from build123d import *

# Parameters (mm, degrees)
SKETCH1_R             = 20
SKETCH1_R_2           = 15
BOSS_EXTRUDE1_DEPTH   = 15
SKETCH1_R_3           = 40
SKETCH1_R_4           = 16
BOSS_EXTRUDE1_2_DEPTH = 15
BOSS_EXTRUDE1_3_DEPTH = 15
SKETCH1_3_R           = 15
BOSS_EXTRUDE2_DEPTH   = 5


with BuildPart() as part:
    # Sketch1 → Boss-Extrude1 (new, symmetric)
    with BuildSketch(Plane.XY):
        with Locations((-70, 0)):
            Circle(SKETCH1_R)
        with Locations((-70, 0)):
            Circle(SKETCH1_R_2, mode=Mode.SUBTRACT)
    extrude(amount=BOSS_EXTRUDE1_DEPTH, both=True)



with BuildPart() as body_2:
    # Sketch1 → Boss-Extrude1 2 (new, symmetric)
    with BuildSketch(Plane.XY):
        Circle(SKETCH1_R_3)
        Circle(SKETCH1_R_4, mode=Mode.SUBTRACT)
        with BuildLine():
            ThreePointArc((26.090759323, 18.527608533), (16, 27.712812921), (3, 31.859064644))
            Line((3, 31.859064644), (3, 20.784609691))
            ThreePointArc((3, 20.784609691), (10.5, 18.186533479), (16.5, 12.990381057))
            Line((16.5, 12.990381057), (26.090759323, 18.527608533))
        make_face(mode=Mode.SUBTRACT)
        with BuildLine():
            ThreePointArc((29.090759323, -13.331456111), (32, 0), (29.090759323, 13.331456111))
            Line((29.090759323, 13.331456111), (19.5, 7.794228634))
            ThreePointArc((19.5, 7.794228634), (21, 0), (19.5, -7.794228634))
            Line((19.5, -7.794228634), (29.090759323, -13.331456111))
        make_face(mode=Mode.SUBTRACT)
        with BuildLine():
            ThreePointArc((3, -31.859064644), (16, -27.712812921), (26.090759323, -18.527608533))
            Line((26.090759323, -18.527608533), (16.5, -12.990381057))
            ThreePointArc((16.5, -12.990381057), (10.5, -18.186533479), (3, -20.784609691))
            Line((3, -20.784609691), (3, -31.859064644))
        make_face(mode=Mode.SUBTRACT)
        with BuildLine():
            ThreePointArc((-26.090759323, -18.527608533), (-16, -27.712812921), (-3, -31.859064644))
            Line((-3, -31.859064644), (-3, -20.784609691))
            ThreePointArc((-3, -20.784609691), (-10.5, -18.186533479), (-16.5, -12.990381057))
            Line((-16.5, -12.990381057), (-26.090759323, -18.527608533))
        make_face(mode=Mode.SUBTRACT)
        with BuildLine():
            ThreePointArc((-29.090759323, 13.331456111), (-32, 0), (-29.090759323, -13.331456111))
            Line((-29.090759323, -13.331456111), (-19.5, -7.794228634))
            ThreePointArc((-19.5, -7.794228634), (-21, 0), (-19.5, 7.794228634))
            Line((-19.5, 7.794228634), (-29.090759323, 13.331456111))
        make_face(mode=Mode.SUBTRACT)
        with BuildLine():
            ThreePointArc((-3, 31.859064644), (-16, 27.712812921), (-26.090759323, 18.527608533))
            Line((-26.090759323, 18.527608533), (-16.5, 12.990381057))
            ThreePointArc((-16.5, 12.990381057), (-10.5, 18.186533479), (-3, 20.784609691))
            Line((-3, 20.784609691), (-3, 31.859064644))
        make_face(mode=Mode.SUBTRACT)
    extrude(amount=BOSS_EXTRUDE1_2_DEPTH, both=True)


with BuildPart() as body_3:
    # Sketch1 → Boss-Extrude1 3 (new, symmetric)
    with BuildSketch(Plane.XY):
        with Locations((70, 0)):
            Circle(SKETCH1_R)
        with Locations((70, 0)):
            Circle(SKETCH1_R_2, mode=Mode.SUBTRACT)
    extrude(amount=BOSS_EXTRUDE1_3_DEPTH, both=True)


with BuildPart() as part_1:
    add(part.part)

    add(body_2.part)  # Boss-Extrude2 merges body 2

    add(body_3.part)  # Boss-Extrude2 merges body 3
    # Sketch1_3 → Boss-Extrude2 (add, symmetric)
    # profile 1 of 2: a face of its own
    with BuildSketch(Plane.XY):
        with BuildLine():
            ThreePointArc((-89.071294105, 6.023764702), (-50, 0), (-89.071294105, -6.023764702))
            Line((-89.071294105, -6.023764702), (-70.02485881, -66.324952937))
            ThreePointArc((-70.02485881, -66.324952937), (-46.6282273, -80.727545655), (-29.002885891, -59.651863383))
            ThreePointArc((-29.002885891, -59.651863383), (-22.168588856, -44.262528341), (-6.003756239, -39.546869801))
            ThreePointArc((-6.003756239, -39.546869801), (-40, 0), (-6.003756239, 39.546869801))
            ThreePointArc((-6.003756239, 39.546869801), (-22.168588856, 44.262528341), (-29.002885891, 59.651863383))
            ThreePointArc((-29.002885891, 59.651863383), (-46.6282273, 80.727545655), (-70.02485881, 66.324952937))
            Line((-70.02485881, 66.324952937), (-89.071294105, 6.023764702))
        make_face()
        with Locations((-50, -60)):
            Circle(SKETCH1_3_R, mode=Mode.SUBTRACT)
        with Locations((-50, 60)):
            Circle(SKETCH1_3_R, mode=Mode.SUBTRACT)
    # profile 2 of 2: a face of its own
    with BuildSketch(Plane.XY):
        with BuildLine():
            ThreePointArc((6.003756239, 39.546869801), (40, 0), (6.003756239, -39.546869801))
            ThreePointArc((6.003756239, -39.546869801), (22.168588856, -44.262528341), (29.002885891, -59.651863383))
            ThreePointArc((29.002885891, -59.651863383), (46.6282273, -80.727545655), (70.02485881, -66.324952937))
            Line((70.02485881, -66.324952937), (89.071294105, -6.023764702))
            ThreePointArc((89.071294105, -6.023764702), (50, 0), (89.071294105, 6.023764702))
            Line((89.071294105, 6.023764702), (70.02485881, 66.324952937))
            ThreePointArc((70.02485881, 66.324952937), (46.6282273, 80.727545655), (29.002885891, 59.651863383))
            ThreePointArc((29.002885891, 59.651863383), (22.168588856, 44.262528341), (6.003756239, 39.546869801))
        make_face()
        with Locations((50, -60)):
            Circle(SKETCH1_3_R, mode=Mode.SUBTRACT)
        with Locations((50, 60)):
            Circle(SKETCH1_3_R, mode=Mode.SUBTRACT)
    extrude(amount=BOSS_EXTRUDE2_DEPTH, both=True)


solid = part_1.part
Source: CAD feature listing. Evaluate the final solid. Frame: model axes, mm. A direction names the side the tool comes from. Coordinates: 2 decimals unless noted, no trailing zeros. Loops run counter-clockwise (first coordinate to the right, second up) from the corner with the lowest first, then second, coordinate; pieces in that order, holes last. Notation, with made-up numbers: (10.5, 65) - (36.5, 65) arc R21 cw to (36.5, 70) - close; hole circle Ø10 at (-37.5, 27). An arc over 180 degrees is marked (long way). One line per item, written item: value. Start each with the question number.
1. Mould query, pull axis Y, two halves, no side actions, for faces 1 (the flat face through (73, 15, 15)), 2 (the cylindrical face through (-21, 0, 0)), 3 (the flat face through (-79.681, -35.752, -0.07)). Classes: pulls with the +Y half, pulls with the -Y half, needs draft (parallel to the pull), parting line crosses it, or undercut.
2. Section B-B (y = -69.5). Return the cut outline in (x, z), and give its area (3 significant figures).
3. Section A-A (x = 0). Return the cut outline in (y, z).
4. Section D-D (y = -47). Return the cut outline in (x, z), and give its area (3 significant figures).
5. Ray query, L1, parallel to Y at x = 50, z = 0.5; L2, parallel to X at y = 25.5, z = -1.5; L3, parallel to Y at x = 52, z = -1.75. Return the intervals inside material, ascending.
6. Contact query for flat-ended pins moving along their axis: P1, Ø5.5, axis at y = -26, z = 0.5, coming from the -X side; P2, Ø2, axis at y = -14, z = -6.5, coming from the +X side; P3, Ø1.5, axis at x = 26.5, y = -49.5, coming from the +Z side; P4, Ø18, axis at x = 70, y = 0, coming from the +Z side. Output: stop coordinate, or through.
7. Set-up query: faces 4 (the flat face through (-21.23, -15.72, 0.21)), 5 (the flat face through (17, 1, -15)), 6 (the flat face through (47, 6, -5)). Return all of +Z, -Z, +X, -X, +Y, -Y with unobstructed straight access to the full face (end or side cutting, diameter ignored); none if empty.
8. Section C-C (y = -25.5). Return the cut outline in (x, z), and give its area (3 significant figures).
Verdict:
1. face 1: needs draft
1. face 2: undercut
1. face 3: pulls with the -Y half
2. outline: (-68.73, -5) - (-61.61, -5) - (-61.61, 5) - (-68.73, 5) - close; (-38.39, -5) - (-31.27, -5) - (-31.27, 5) - (-38.39, 5) - close; (31.27, -5) - (38.39, -5) - (38.39, 5) - (31.27, 5) - close; (61.61, -5) - (68.73, -5) - (68.73, 5) - (61.61, 5) - close
2. area: 285 mm2
3. outline: (-40, -15) - (-16, -15) - (-16, 15) - (-40, 15) - close; (16, -15) - (40, -15) - (40, 15) - (16, 15) - close
4. outline: (-76.13, -5) - (-57.48, -5) - (-57.48, 5) - (-76.13, 5) - close; (-42.52, -5) - (-24.76, -5) - (-24.76, 5) - (-42.52, 5) - close; (24.76, -5) - (42.52, -5) - (42.52, 5) - (24.76, 5) - close; (57.48, -5) - (76.13, -5) - (76.13, 5) - (57.48, 5) - close
4. area: 728 mm2
5. L1: y = -81 to -75, -45 to 45, 75 to 81
5. L2: x = -82.92 to -19.33, -3 to 3, 19.33 to 82.92
5. L3: y = -80.9 to -74.87, -45.13 to 45.13, 74.87 to 80.9
6. P1: stops at x = -83.63
6. P2: stops at x = 85.2
6. P3: stops at z = 5
6. P4: passes through
7. face 4: +Z, -Z
7. face 5: -Z, +X, -X, +Y, -Y
7. face 6: -Z
8. outline: (-82.92, -5) - (-30.82, -5) - (-30.82, -15) - (-19.33, -15) - (-19.33, 15) - (-30.82, 15) - (-30.82, 5) - (-82.92, 5) - close; (-3, -15) - (3, -15) - (3, 15) - (-3, 15) - close; (19.33, -15) - (30.82, -15) - (30.82, -5) - (82.92, -5) - (82.92, 5) - (30.82, 5) - (30.82, 15) - (19.33, 15) - close
8. area: 1,910 mm2
